```python
from build123d import *

# Parameters (mm, degrees)
CROQUIS1_R              = 75
SALIENTE_EXTRUIR1_DEPTH = 8
CROQUIS2_R              = 3.97
CORTAR_EXTRUIR1_DEPTH   = 20
SALIENTE_EXTRUIR2_DEPTH = 10
SALIENTE_EXTRUIR3_DEPTH = 22
CROQUIS5_R              = 15
CORTAR_EXTRUIR2_DEPTH   = 12
CROQUIS6_R              = 5
CORTAR_EXTRUIR3_DEPTH   = 126
CROQUIS7_R              = 15
SALIENTE_EXTRUIR4_DEPTH = 68
CROQUIS8_R              = 75
SALIENTE_EXTRUIR5_DEPTH = 8
CROQUIS9_R              = 15
CROQUIS9_R_2            = 13
SALIENTE_EXTRUIR6_DEPTH = 18


with BuildPart() as part:
    # Croquis1 → Saliente-Extruir1 (new body)
    with BuildSketch(Plane(origin=(0, 0, 0), x_dir=(1, 0, 0), z_dir=(0, 1, 0))):
        Circle(CROQUIS1_R)
    extrude(amount=SALIENTE_EXTRUIR1_DEPTH)

    # Croquis2 → Cortar-Extruir1 (cut)
    with BuildSketch(Plane(origin=(0, 8, 0), x_dir=(1, 0, 0), z_dir=(0, 1, 0))):
        with Locations((0, 63)):
            Circle(CROQUIS2_R)
        with Locations((63, 0)):
            Circle(CROQUIS2_R)
        with Locations((0, -63)):
            Circle(CROQUIS2_R)
        with Locations((-63, 0)):
            Circle(CROQUIS2_R)
    extrude(amount=-CORTAR_EXTRUIR1_DEPTH, mode=Mode.SUBTRACT)

    # Croquis3 → Saliente-Extruir2 (add)
    with BuildSketch(Plane(origin=(0, 8, 0), x_dir=(1, 0, 0), z_dir=(0, 1, 0))):
        Polygon((-55, 0), (-55, 30), (55, 30), (55, 0), (55, -30), (-55, -30), align=None)
    extrude(amount=SALIENTE_EXTRUIR2_DEPTH)

    # Croquis4 → Saliente-Extruir3 (add)
    with BuildSketch(Plane(origin=(55, 0, 0), x_dir=(0, 0, -1), z_dir=(1, 0, 0))):
        with BuildLine():
            Line((-30, 18), (30, 18))
            Line((30, 18), (19.464281728, 62.598174498))
            ThreePointArc((19.464281728, 62.598174498), (0, 78.000036798), (-19.464281728, 62.598174498))
            Line((-19.464281728, 62.598174498), (-30, 18))
        make_face()
    saliente_extruir3 = extrude(amount=-SALIENTE_EXTRUIR3_DEPTH)

    # Simetría1: Saliente-Extruir3 across plane
    add(saliente_extruir3.mirror(Plane(origin=(0, 0, 0), x_dir=(0, 0, 1), z_dir=(1, 0, 0))))

    # Croquis5 → Cortar-Extruir2 (cut)
    with BuildSketch(Plane.ZY.offset(55)):
        with Locations((0, 58)):
            Circle(CROQUIS5_R)
    cortar_extruir2 = extrude(amount=-CORTAR_EXTRUIR2_DEPTH, mode=Mode.SUBTRACT)

    # Simetría2: Cortar-Extruir2 across plane
    add(cortar_extruir2.mirror(Plane(origin=(0, 0, 0), x_dir=(0, 0, 1), z_dir=(1, 0, 0))), mode=Mode.SUBTRACT)

    # Croquis6 → Cortar-Extruir3 (cut)
    with BuildSketch(Plane.ZY.offset(43)):
        with Locations((0, 58)):
            Circle(CROQUIS6_R)
    extrude(amount=-CORTAR_EXTRUIR3_DEPTH, mode=Mode.SUBTRACT)

    # Croquis7 → Saliente-Extruir4 (add)
    with BuildSketch(Plane.ZY.offset(55)):
        with BuildLine():
            Line((-19.464281728, 62.598174498), (-28.151527476, 25.824668242))
            Line((-28.151527476, 25.824668242), (28.151527476, 25.824668242))
            Line((28.151527476, 25.824668242), (19.464281728, 62.598174498))
            ThreePointArc((19.464281728, 62.598174498), (0, 78.000036798), (-19.464281728, 62.598174498))
        make_face()
        with Locations((0, 58)):
            Circle(CROQUIS7_R, mode=Mode.SUBTRACT)
    extrude(amount=SALIENTE_EXTRUIR4_DEPTH)

    # Croquis8 → Saliente-Extruir5 (add)
    with BuildSketch(Plane.XZ):
        Circle(CROQUIS8_R)
    extrude(amount=SALIENTE_EXTRUIR5_DEPTH)

    # Croquis9 → Saliente-Extruir6 (add)
    with BuildSketch(Plane.XZ.offset(8)):
        Circle(CROQUIS9_R)
        Circle(CROQUIS9_R_2, mode=Mode.SUBTRACT)
    extrude(amount=SALIENTE_EXTRUIR6_DEPTH)


solid = part.part
```
Verification items for the finished model (mm, model axes). A direction names the side the tool comes from. Coordinates: 2 decimals unless noted, no trailing zeros. Loops run counter-clockwise (first coordinate to the right, second up) from the corner with the lowest first, then second, coordinate; pieces in that order, holes last. Notation, with made-up numbers: (-32.5, -39) - (-21.5, -39) arc R11 cw to (-21.5, -19) - close; hole circle Ø4 at (83, 55). An arc over 180 degrees is marked (long way). Answer as a JSON object with one key per item and string values.
(1) Go/stop test with flat-tipped pins: pin 1 Ø1 at (x, z) = (0.5, -16.5) entering from +Y; pin 2 Ø9 at (y, z) = (62, 5) entering from -X; pin 3 Ø10.5 at (x, z) = (-63, 0) entering from -Y. Record where each tip stops, or that it passes through.
Response:
{"pin 1": "stops at y = 18", "pin 2": "stops at x = -43", "pin 3": "stops at y = -8"}
(2) Access from +Z, -Z, +X, -X, +Y, -Y to the whole of each face (thin tool, end or side, straight path). Record for faces 4 (the flat face through (0, -8, 0)), 5 (the flat face through (-1, 13, -30)), 6 (the flat face through (55, 36, 0)), 7 (the cylindrical face through (49.084, 43.357, -3.252)).
Response:
{"face 4": "-Y", "face 5": "-Z, +X, -X, +Y", "face 6": "+Z, -Z, +X, +Y", "face 7": "+X"}
(3) Scan lines: line 1 along Z through (x, y) = (0, 2); line 2 along Y through (x, z) = (46.5, 0); line 3 along X through (y, z) = (58, -17). Record each from-to range of solid material in increasing order.
Response:
{"line 1": "z = -75 to -66.97, -59.03 to 59.03, 66.97 to 75", "line 2": "y = -8 to 43, 73 to 78", "line 3": "x = -123 to -33, 33 to 55"}
(4) Mould release check, pull along Y, two halves, no side actions. Record for faces 1 (the flat face through (-33, 42, 0)), 2 (the flat face through (-43, 62, -4)), 3 (the flat face through (0, 18, 0)): pulls with the +Y half, pulls with the -Y half, needs draft (parallel to the pull), parting line crosses it, or undercut.
Response:
{"face 1": "needs draft", "face 2": "undercut", "face 3": "pulls with the +Y half"}
(5) Cross-section at C-C, the plane x = -63. Record the boundary of the cut face in (y, z), then the cut area to 3 significant figures.
Response:
{"outline": "(-8, -40.69) - (8, -40.69) - (8, -3.97) - (0, -3.97) - (0, 3.97) - (8, 3.97) - (8, 40.69) - (-8, 40.69) - close; (25.82, -28.15) - (62.6, -19.46) arc R20 ccw to (62.6, 19.46) - (25.82, 28.15) - close; hole circle Ø30 at (58, 0)", "area": "2,730 mm²"}
(6) Cross-section at A-A, the plane y = 38.5. Record the boundary of the cut face in (x, z), then the cut area to 3 significant figures.
Response:
{"outline": "(-123, -25.16) - (-33, -25.16) - (-33, 25.16) - (-123, 25.16) - close; (33, -25.16) - (55, -25.16) - (55, 25.16) - (33, 25.16) - close", "area": "5,640 mm²"}
(7) Cross-section at B-B, the plane x = -108. Record the boundary of the cut face in (y, z).
Response:
{"outline": "(25.82, -28.15) - (62.6, -19.46) arc R20 ccw to (62.6, 19.46) - (25.82, 28.15) - close; hole circle Ø30 at (58, 0)"}
